from build123d import *

# Parameters (mm, degrees)
SKETCH1_W             = 220
SKETCH1_H             = 220
BOSS_EXTRUDE1_DEPTH   = 3.175
M3X0_5_TAPPED_HOLE1_D = 2.5
SKETCH4_R             = 2.75
CUT_EXTRUDE1_DEPTH    = 4.175
CUT_EXTRUDE2_DEPTH    = 4.175


with BuildPart() as part:
    # Sketch1 → Boss-Extrude1 (new body)
    with BuildSketch(Plane(origin=(0, 0, 0), x_dir=(1, 0, 0), z_dir=(0, 1, 0))):
        Rectangle(SKETCH1_W, SKETCH1_H)
    extrude(amount=BOSS_EXTRUDE1_DEPTH)

    # M3x0.5 Tapped Hole1 (through all)
    with Locations(Plane(origin=(0, 3.175, 0), x_dir=(-1, 0, 0), z_dir=(0, 1, 0))):
        with Locations((104.5, -104.5), (-104.5, -104.5), (-104.5, 104.5), (104.5, 104.5)):
            Hole(M3X0_5_TAPPED_HOLE1_D / 2)

    # Sketch4 → Cut-Extrude1 (cut, through all)
    with BuildSketch(Plane(origin=(0, 3.175, 0), x_dir=(1, 0, 0), z_dir=(0, 1, 0))):
        with Locations(Location((-70, 38, 0), (0, 0, 270))):  # turned: the seam where the file's is
            Circle(SKETCH4_R)
        with Locations(Location((-70, -38, 0), (0, 0, 270))):  # turned: the seam where the file's is
            Circle(SKETCH4_R)
        with Locations(Location((70, -38, 0), (0, 0, 270))):  # turned: the seam where the file's is
            Circle(SKETCH4_R)
        with Locations(Location((70, 38, 0), (0, 0, 270))):  # turned: the seam where the file's is
            Circle(SKETCH4_R)
    extrude(amount=-CUT_EXTRUDE1_DEPTH, mode=Mode.SUBTRACT)

    # Sketch5 → Cut-Extrude2 (cut, through all)
    with BuildSketch(Plane(origin=(0, 3.175, 0), x_dir=(1, 0, 0), z_dir=(0, 1, 0))):
        with BuildLine():
            Line((-110, 102.928932188), (-110, -102.928932188))
            Line((-110, -102.928932188), (-101.859871939, -94.788804128))
            ThreePointArc((-101.859871939, -94.788804128), (-100.483364969, -92.728715863), (-100, -90.298676067))
            Line((-100, -90.298676067), (-100, 90.298676067))
            ThreePointArc((-100, 90.298676067), (-100.483364969, 92.728715863), (-101.859871939, 94.788804128))
            Line((-101.859871939, 94.788804128), (-110, 102.928932188))
        make_face()
        with BuildLine():
            Line((110, 102.928932188), (101.859871939, 94.788804128))
            ThreePointArc((101.859871939, 94.788804128), (100.483364969, 92.728715863), (100, 90.298676067))
            Line((100, 90.298676067), (100, -90.298676067))
            ThreePointArc((100, -90.298676067), (100.483364969, -92.728715863), (101.859871939, -94.788804128))
            Line((101.859871939, -94.788804128), (110, -102.928932188))
            Line((110, -102.928932188), (110, 102.928932188))
        make_face()
    extrude(amount=-CUT_EXTRUDE2_DEPTH, mode=Mode.SUBTRACT)


solid = part.part
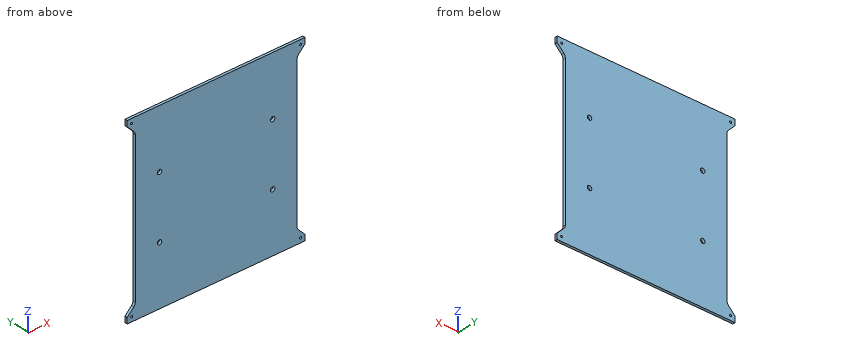
Input: part model. Units: mm. Frame: model coordinates. Give positions to 0.01 mm unless a question says otherwise; leave off trailing zeros. Write each loop counter-clockwise with the first axis right and the second up, starting at its lowest first coordinate (ties: lowest second). Pieces come first, ordered by that corner, then holes. Notation, with made-up numbers: (63, -22.5) -> (86, -22.5) arc R30 ccw to (86, 7.5) -> close; hole circle Ø7 at (59, -7). An arc over 180 degrees is marked (long way). Use one line per item in the form item = value. Start each with the question number.
1) Section query A-A on x = -70. Return the cut outline in (y, z) (3 decimals), then the cut area to 3 significant figures.
2) Ray query, probe 1 along X at (y, z) = (0.9, 104.5); probe 2 along X at (y, z) = (2.15, -38); probe 3 along Z at (x, y) = (-104.5, 2.55). Return the intervals inside material, ascending. Write a range as from..to.
3) Section query C-C on y = 2.4. Count the separate pieces of the cut face and the enclosed holes in it, then the cut area to 3 significant figures.
4) Pin query (flat end, axial travel): pin 1 (4.5 mm diameter, centred on x = -70, z = 38, fed in from -Y); pin 2 (1.6 mm diameter, centred on y = 1.5, z = -1, fed in from +X); pin 3 (1.6 mm diameter, centred on y = 2, z = -38.5, fed in from -X). Return the tip coordinate at first contact, or that it passes through.
5) Section query B-B on z = -38. Return the cut outline in (x, y) (3 decimals), then the cut area to 3 significant figures.
Outcome:
q1.outline = (0, -110) -> (3.175, -110) -> (3.175, -40.75) -> (0, -40.75) -> close; (0, -35.25) -> (3.175, -35.25) -> (3.175, 35.25) -> (0, 35.25) -> close; (0, 40.75) -> (3.175, 40.75) -> (3.175, 110) -> (0, 110) -> close
q1.area = 664 mm^2
q2.probe_1 = -110..-105.75, -103.25..103.25, 105.75..110
q2.probe_2 = -100..-72.75, -67.25..67.25, 72.75..100
q2.probe_3 = -110..-105.75, -103.25..-97.43, 97.43..103.25, 105.75..110
q3.separate_pieces = 1
q3.enclosed_holes = 8
q3.area = 44,400 mm^2
q4.pin_1 = through
q4.pin_2 = 100
q4.pin_3 = -100
q5.outline = (-100, 0) -> (-72.75, 0) -> (-72.75, 3.175) -> (-100, 3.175) -> close; (-67.25, 0) -> (67.25, 0) -> (67.25, 3.175) -> (-67.25, 3.175) -> close; (72.75, 0) -> (100, 0) -> (100, 3.175) -> (72.75, 3.175) -> close
q5.area = 600 mm^2
